```python
from build123d import *

# Parameters (mm, degrees)
F0_W      = 114.3
F0_H      = 38.1
F2_DEPTH  = 25.4
F1_W      = 60.96
F1_H      = 38.1
F3_DEPTH  = 38.1
F5_DEPTH  = 25.4
F6_W      = 25.4
F6_H      = 19.05
F7_DEPTH  = 228.6
F8_W      = 12.7
F8_H      = 177.8
F9_DEPTH  = 7.62
F10_W     = 6.35
F10_H     = 165.1
F11_DEPTH = 11.431
F13_DEPTH = 6.35
F14_R     = 5.08


with BuildPart() as f2:
    # F0 (on Top) → F2 (new body, symmetric)
    with BuildSketch(Plane.XY):
        Rectangle(F0_W, F0_H)
    extrude(amount=F2_DEPTH, both=True)

    # F1 (on face) → F3 (cut, symmetric)
    with BuildSketch(Plane.XY):
        with Locations((0, -12.7)):
            Rectangle(F1_W, F1_H)
    extrude(amount=F3_DEPTH, both=True, mode=Mode.SUBTRACT)

    # F4 (on Top) → F5 (join, symmetric)
    with BuildSketch(Plane.XY):
        Polygon((-26.9186757505, 0), (-30.5502526462, 4.3267654255), (-30.6185223162, -6.3184089959), align=None)
    extrude(amount=F5_DEPTH, both=True)

    # F6 (on face) → F7 (join)
    with BuildSketch(Plane(origin=(0, 19.05, 0), x_dir=(-1, 0, 0), z_dir=(0, 1, 0))):
        with Locations((44.45, 15.875)):
            Rectangle(F6_W, F6_H)
    extrude(amount=F7_DEPTH)

    # F8 (on face) → F9 (cut)
    with BuildSketch(Plane(origin=(0, 0, 6.35), x_dir=(1, 0, 0), z_dir=(0, 0, -1))):
        with Locations((-44.45, -152.4)):
            Rectangle(F8_W, F8_H)
    extrude(amount=-F9_DEPTH, mode=Mode.SUBTRACT)

    # F10 (on face) → F11 (cut, through all)
    with BuildSketch(Plane(origin=(0, 0, 13.97), x_dir=(1, 0, 0), z_dir=(0, 0, -1))):
        with Locations((-44.45, -152.4)):
            Rectangle(F10_W, F10_H)
    extrude(amount=-F11_DEPTH, mode=Mode.SUBTRACT)

    # F12 (on face) → F13 (join)
    with BuildSketch(Plane.XY.offset(25.4)):
        Polygon((0, 19.05), (-31.75, 61.1579380929), (-31.75, 19.05), align=None)
    extrude(amount=-F13_DEPTH)

    # F14
    f14_edges = [f2.edges().sort_by_distance(p)[0] for p in [
        (28.575, 19.05, 25.4),
        (57.15, 19.05, 0),
        (0, 19.05, -25.4),
        (-57.15, 19.05, -9.525),
        (-57.15, 0, -25.4),
        (-30.48, -12.565924, -25.4),
        (-57.15, -19.05, 0),
        (57.15, 0, 25.4),
        (57.15, 0, -25.4),
        (30.48, -6.35, 25.4),
        (57.15, -19.05, 0),
        (43.815, -19.05, 25.4),
        (30.48, -19.05, 0),
        (43.815, -19.05, -25.4),
        (0, 6.35, 25.4),
        (-30.48, 5.296532, 25.4),
        (-30.48, -12.565924, 25.4),
        (-30.48, -19.05, 0),
        (-43.815, -19.05, -25.4),
        (-43.815, -19.05, 25.4),
        (30.48, -6.35, -25.4),
        (-26.918676, 0, 0),
        (-28.699338, 2.121532, 25.4),
        (-30.48, -6.081848, 0),
        (-28.699338, -3.040924, 25.4),
        (0, 6.35, -25.4),
        (-28.699338, -3.040924, -25.4),
        (-28.699338, 2.121532, -25.4),
        (-30.48, 5.296532, -25.4),
    ]]
    fillet(f14_edges, radius=F14_R)


solid = f2.part
```
Geometry check sheet. Reference: the model listing, model coordinates, mm. A direction names the side the tool comes from. Round coordinates to 2 decimals unless told otherwise and drop trailing zeros. Write each loop counter-clockwise with the first axis right and the second up, starting at its lowest first coordinate (ties: lowest second). Pieces come first, ordered by that corner, then holes. Notation, with made-up numbers: (49.25, 0.5) - (108.25, 0.5) arc R21 ccw to (108.25, 27.5) - close; hole circle Ø8 at (51, 33.25). An arc over 180 degrees is marked (long way). Write each question's results on one line, items separated by ' | '.
(1) Set-up check for faces 1 (the face through (-32.008, -10.669, 23.951)), 2 (the face through (-31.88, 2.48, 24.51)), 3 (the face through (-45, 241.3, 10)): record each of +Z, -Z, +X, -X, +Y, -Y from which the full face is reachable in a straight line by a thin tool's end or side.
Computed:
face 1: +Z, -Y | face 2: +Z | face 3: -Z
(2) Sectioned sample at A-A, the plane y = 113. Enter the section's corners in (x, z) (3 decimals).
Computed:
outline: (-57.15, 6.35) - (-50.8, 6.35) - (-50.8, 13.97) - (-47.625, 13.97) - (-47.625, 25.4) - (-57.15, 25.4) - close; (-41.275, 13.97) - (-38.1, 13.97) - (-38.1, 6.35) - (-31.75, 6.35) - (-31.75, 25.4) - (-41.275, 25.4) - close
(3) Thickness scan on probe 1 along X at (y, z) = (223, 10); probe 2 along Y at (x, z) = (35, 15); probe 3 along Y at (x, z) = (-9, 8). Record the ranges inside material, lowest first. Write a range as from..to.
Computed:
probe 1: x = -57.15..-50.8, -38.1..-31.75 | probe 2: y = -19.02..19.05 | probe 3: y = 6.35..19.05
(4) Sectioned sample at D-D, the plane y = 39.5. Enter the section's corners in (x, z).
Computed:
outline: (-57.15, 6.35) - (-31.75, 6.35) - (-31.75, 19.05) - (-15.42, 19.05) - (-15.42, 25.4) - (-57.15, 25.4) - close
(5) Depth check by flat-ended pin: pin 1 Ø6 at (x, z) = (-24.5, 6) entering from -Y; pin 2 Ø2.5 at (y, z) = (174, 10.5) entering from +X; pin 3 Ø7.5 at (x, y) = (-46.5, 153.5) entering from -Z. Enter the tip coordinate at first touch or a pass-through.
Computed:
pin 1: stops at y = 6.35 | pin 2: stops at x = -31.75 | pin 3: stops at z = 13.97
(6) Sectioned sample at C-C, the plane z = 3.5. Enter the section's corners in (x, y).
Computed:
outline: (-57.15, -13.97) arc R5.08 ccw to (-52.07, -19.05) - (-35.56, -19.05) arc R5.08 ccw to (-30.48, -13.97) - (-30.48, -7.46) arc R5.08 cw to (-29.78, -4.89) - (-28.73, -3.09) arc R5.08 ccw to (-29.22, 2.74) - (-30.48, 4.24) - (-30.48, 6.35) - (30.48, 6.35) - (30.48, -13.97) arc R5.08 ccw to (35.56, -19.05) - (52.07, -19.05) arc R5.08 ccw to (57.15, -13.97) - (57.15, 13.97) arc R5.08 ccw to (52.07, 19.05) - (-52.07, 19.05) arc R5.08 ccw to (-57.15, 13.97) - close
(7) Draft check along X on faces 4 (the face through (26.399, 17.601, 23.872)), 5 (the face through (-38.1, 154, 10)), 6 (the face through (55.622, 17.601, -0.284)), 7 (the face through (-49, 151, 13.97)). Enter one of: pulls with the +X half, pulls with the -X half, needs draft (parallel to the pull), parting line crosses it, or undercut.
Computed:
face 4: needs draft | face 5: undercut | face 6: pulls with the +X half | face 7: undercut
(8) Sectioned sample at B-B, the plane x = 38.5. Enter the section's corners in (y, z), plus the area to 3 significant figures.
Computed:
outline: (-19.05, -20.32) arc R5.08 ccw to (-13.97, -25.4) - (13.97, -25.4) arc R5.08 ccw to (19.05, -20.32) - (19.05, 20.32) arc R5.08 ccw to (13.97, 25.4) - (-13.97, 25.4) arc R5.08 ccw to (-19.05, 20.32) - close | area: 1,910 mm^2
